The model under review builds one solid part; all positions refer to its coordinate system, in mm. Give positions to 0.01 mm unless a question says otherwise; leave off trailing zeros. Order: outer loops, then holes, each group sorted by start corner. A loop starts at its lowest first (then second) coordinate and runs counter-clockwise, first axis right, second up. Notation, with made-up numbers: (-32, 86.5) -> (18, 86.5) arc R18 cw to (18, 107.5) -> close; hole circle Ø10 at (-5, 26.5). An arc over 180 degrees is marked (long way). Use one line per item in the form item = value.
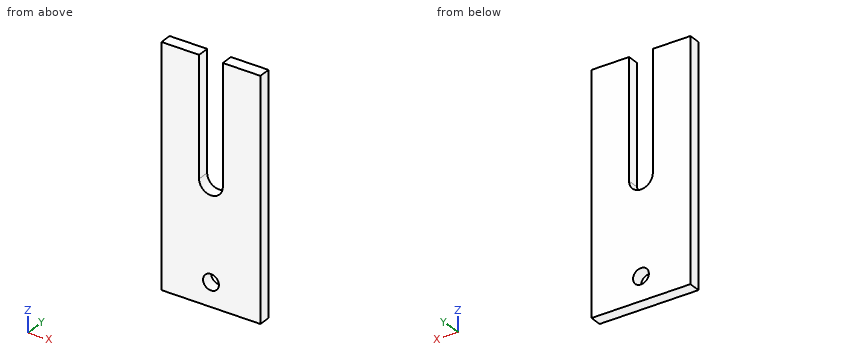
Autodesk Inventor part; units mm, degrees
ref_plane "YZ Plane" through (0, 0, 0) normal (1, 0, 0) x (0, 1, 0)
ref_plane "XZ Plane" through (0, 0, 0) normal (0, 1, 0) x (-1, 0, 0)
ref_plane "XY Plane" through (0, 0, 0) normal (0, 0, 1) x (1, 0, 0)
sketch "Sketch1" plane through (0, 0, 0) normal (0, 1, 0) x (-1, 0, 0)
  line L0 (0, 0) -> (25, 0)
  line L1 (25, 0) -> (25, -60)
  line L2 (25, -60) -> (0, -60)
  line L3 (0, -60) -> (0, 0)
  point P0 (12.5, -54)
  dimension "d0" = 25
  dimension "d1" = 60
  dimension "d15" = 6
extrude "Extrusion1" add sketch "Sketch1" along normal blind 3
sketch "Sketch2" plane through (0, 0, 0) normal (0, -1, 0) x (1, 0, 0)
  point P0 (0, 0)
  point P1 (-12.5, -54)
hole "Hole2" at (-12.5, 0, -54) direction (0, 1, 0) diameter 4 end through all
sketch "Sketch3" plane through (0, 0, 0) normal (0, -1, 0) x (1, 0, 0)
  point P0 (0, 0)
  point P1 (-12.5, -30)
hole "Hole3" at (-12.5, 0, -30) direction (0, 1, 0) diameter 6 end through all
sketch "Sketch4" plane through (0, 0, 0) normal (0, -1, 0) x (1, 0, 0)
  circle A0 centre (-12.5, -30) radius 3
  line L0 (-25, 0) -> (0, 0)
  line L1 (-9.5, -30) -> (-15.5, -30)
  line L2 (-15.5, -30) -> (-15.5, 0)
  line L3 (-15.5, 0) -> (-9.5, 0)
  line L4 (-9.5, 0) -> (-9.5, -30)
extrude "Extrusion2" cut sketch "Sketch4" against normal through all contours L1 A0 | A0 L2 L0 L4 picked at (-11.666, -28.6328)
properties part number "Spacer_lazy_susan"
1. For pin 1 Ø2.5 at (x, z) = (-12.5, -54) entering from -Y; pin 2 Ø2 at (x, z) = (-13, -49) entering from -Y, all flat-tipped, find the tip position at first contact; note any pin that passes through.
Values:
pin_1 = through
pin_2 = 0
2. For L1, parallel to Z at x = -12.5, y = 2; L2, parallel to X at y = 2.1, z = -25; L3, parallel to X at y = 0.7, z = -54, list the stretches that pass through material, from the lowest coordinate up.
Values:
L1 = -60 to -56, -52 to -33
L2 = -25 to -15.5, -9.5 to 0
L3 = -25 to -14.5, -10.5 to 0
3. Add section B-B on x = -12.5. Give the boundary of the cut face in (y, z), then the cut area to 3 significant figures.
Values:
outline = (0, -60) -> (3, -60) -> (3, -56) -> (0, -56) -> close; (0, -52) -> (3, -52) -> (3, -33) -> (0, -33) -> close
area = 69.0 mm^2
4. Add section A-A on z = -54. Give the boundary of the cut face in (x, y), then the cut area to 3 significant figures.
Values:
outline = (-25, 0) -> (-14.5, 0) -> (-14.5, 3) -> (-25, 3) -> close; (-10.5, 0) -> (0, 0) -> (0, 3) -> (-10.5, 3) -> close
area = 63.0 mm^2
5. Add section C-C on y = 2.2. Give the boundary of the cut face in (x, z), then the cut area to 3 significant figures.
Values:
outline = (-25, -60) -> (0, -60) -> (0, 0) -> (-9.5, 0) -> (-9.5, -30) arc R3 cw to (-15.5, -30) -> (-15.5, 0) -> (-25, 0) -> close; hole circle Ø4 at (-12.5, -54)
area = 1,290 mm^2
